The figure shows three views and two pictorial views of one solid part (mm, origin at its lowest corner). Answer the questions. A direction names the side the tool comes from. Give positions to 0.01 mm unless a question says otherwise; leave off trailing zeros. Loops run counter-clockwise (first coordinate to the right, second up) from the corner with the lowest first, then second, coordinate; pieces in that order, holes last. Notation, with made-up numbers: (6.25, -30.5) - (32.25, -30.5) arc R33 cw to (32.25, 1.5) - close; hole circle Ø3 at (85.5, 12). An arc over 180 degrees is marked (long way). Write item = value, one per line.
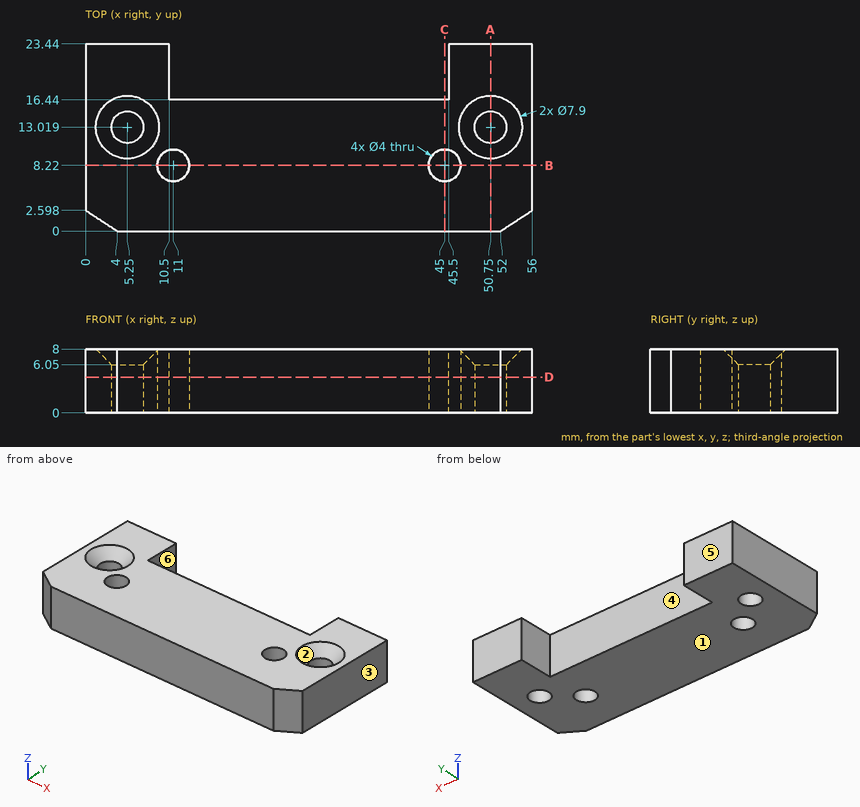
1) A cutting plane is placed at A-A on x = 50.75. Determine the outline of the cut face in (y, z), then the cut area to 3 significant figures.
Output:
outline = (0, 0) - (11.02, 0) - (11.02, 6.05) - (9.07, 8) - (0, 8) - close; (15.02, 0) - (23.44, 0) - (23.44, 8) - (16.97, 8) - (15.02, 6.05) - close
area = 152 mm²
2) A cutting plane is placed at B-B on y = 8.22. Determine the outline of the cut face in (x, z), then the cut area to 3 significant figures.
Output:
outline = (0, 0) - (9, 0) - (9, 8) - (0, 8) - close; (13, 0) - (43, 0) - (43, 8) - (13, 8) - close; (47, 0) - (56, 0) - (56, 8) - (47, 8) - close
area = 384 mm²
3) Each of these flat-tipped pins is pushed along its axis until it touches: P1, Ø4, axis at x = 42.5, y = 19, coming from the +Z side; P2, Ø5, axis at x = 50.75, y = 13.02, coming from the -Z side; P3, Ø6.5, axis at x = 5.25, y = 13.02, coming from the +Z side; P4, Ø1.5, axis at x = 39, z = 1, coming from the +Y side. Where does it stop, or does it pass through?
Output:
P1 = through
P2 = 0
P3 = 7.3
P4 = 16.44
4) A cutting plane is placed at C-C on x = 45. Determine the outline of the cut face in (y, z).
Output:
outline = (0, 0) - (6.22, 0) - (6.22, 8) - (0, 8) - close; (10.22, 0) - (16.44, 0) - (16.44, 8) - (10.22, 8) - close
5) A tool of negligible diameter and unlimited length cuts with its end or side. For the marked faces 5 and 6, from which of +Z, -Z, +X, -X, +Y, -Y can it reach the whole face along a straight path? Write none if from no direction.
Output:
face_5 = +Z, -Z, +X, -X, +Y
face_6 = +Z, -Z, +Y
6) Find the intervals of material crossed by probe 1 along X at (y, z) = (8.22, 2.75); probe 2 along X at (y, z) = (6.5, 7.5); probe 3 along X at (y, z) = (19, 7.75), in increasing order.
Output:
probe_1 = 0 to 9, 13 to 43, 47 to 56
probe_2 = 0 to 9.98, 12.02 to 43.98, 46.02 to 56
probe_3 = 0 to 10.5, 45.5 to 56
7) The mould has two halves that part along X. Classify the marked faces 1, 2, 3 and 4: pulls with the +X half, pulls with the -X half, needs draft (parallel to the pull), parting line crosses it, or undercut.
Output:
face_1 = needs draft
face_2 = undercut
face_3 = pulls with the +X half
face_4 = undercut
8) A cutting plane is placed at D-D on z = 4.5. Determine the outline of the cut face in (x, y), then the cut area to 3 significant figures.
Output:
outline = (0, 2.6) - (4, 0) - (52, 0) - (56, 2.6) - (56, 23.44) - (45.5, 23.44) - (45.5, 16.44) - (10.5, 16.44) - (10.5, 23.44) - (0, 23.44) - close; hole circle Ø4 at (5.25, 13.02); hole circle Ø4 at (11, 8.22); hole circle Ø4 at (45, 8.22); hole circle Ø4 at (50.75, 13.02)
area = 1,010 mm²
